from build123d import *

# Parameters (mm, degrees)
SKETCH_1_R               = 3
SKETCH_1_R_2             = 1.40625
EXTRUDE_1_DEPTH          = 5
CUT_EXTRUDE_2_DEPTH      = 7.557438524
PATTERN_CIRCULAR_1_COUNT = 7


with BuildPart() as part:
    # 草图1 → 凸台-拉伸1 (new body)
    with BuildSketch(Plane.XY):
        Circle(SKETCH_1_R)
        Circle(SKETCH_1_R_2, mode=Mode.SUBTRACT)
    extrude(amount=EXTRUDE_1_DEPTH)

    # 草图1<3> → 切除-拉伸2 (cut, through all)
    with BuildSketch(Plane.XY):
        with BuildLine():
            Line((1.546319716, 0.559598866), (1.322324253, 0.478536971))
            ThreePointArc((1.322324253, 0.478536971), (1.385109661, 0.242920339), (1.40625, 0))
            ThreePointArc((1.40625, 0), (1.385109661, -0.242920339), (1.322324253, -0.478536971))
            Line((1.322324253, -0.478536971), (1.546319716, -0.559598866))
            add(Edge.make_bspline(
                [(1.546319716, -0.559598866), (1.558105463, -0.563864019), (1.591921474, -0.573215837), (1.658734166, -0.580959295), (1.767731952, -0.57845396), (1.907008009, -0.553308364), (2.079413065, -0.496026363), (2.261035814, -0.40341458), (2.393734523, -0.311147352), (2.48335867, -0.236539754), (2.523284743, -0.200650618)],
                knots=[0, 0, 0, 0, 0, 0.005604068, 0.015718248, 0.029959916, 0.048733667, 0.068727063, 0.096888892, 0.120945025, 0.120945025, 0.120945025, 0.120945025, 0.120945025], degree=4))
            ThreePointArc((2.523284743, -0.200650618), (2.529257902, -0.100404327), (2.53125, 0))
            ThreePointArc((2.53125, 0), (2.529257902, 0.100404327), (2.523284743, 0.200650618))
            add(Edge.make_bspline(
                [(1.546319716, 0.559598866), (1.558105463, 0.563864019), (1.591921474, 0.573215837), (1.658734166, 0.580959295), (1.767731952, 0.57845396), (1.907008009, 0.553308364), (2.079413065, 0.496026363), (2.261035814, 0.40341458), (2.393734523, 0.311147352), (2.48335867, 0.236539754), (2.523284743, 0.200650618)],
                knots=[0, 0, 0, 0, 0, 0.005604068, 0.015718248, 0.029959916, 0.048733667, 0.068727063, 0.096888892, 0.120945025, 0.120945025, 0.120945025, 0.120945025, 0.120945025], degree=4))
        make_face()
    cut_extrude_2 = extrude(amount=CUT_EXTRUDE_2_DEPTH, mode=Mode.SUBTRACT)

    # 阵列(圆周)1: 切除-拉伸2 ×7 about axis
    pattern_circular_1_axis = Axis((0, 0, 5), (0, 0, 1))
    for i in range(1, PATTERN_CIRCULAR_1_COUNT):
        add(cut_extrude_2.rotate(pattern_circular_1_axis, i * 360 / PATTERN_CIRCULAR_1_COUNT), mode=Mode.SUBTRACT)


solid = part.part
Geometry check sheet. Reference: the model listing, model coordinates, mm. Coordinates: 2 decimals unless noted, no trailing zeros. Order: outer loops, then holes, each group sorted by start corner. A loop starts at its lowest first (then second) coordinate and runs counter-clockwise, first axis right, second up. Notation, with made-up numbers: (18.25, -20.5) -> (41.25, -20.5) arc R14 cw to (41.25, -14.5) -> close; hole circle Ø6 at (-1.75, 33). An arc over 180 degrees is marked (long way). Use a Markdown table: item, result. Add a question column.
1. Cross-section at C-C (x = 2.75). Enter the section's corners in (y, z), and give its area (3 significant figures).
2. Go/stop test with flat-tipped pins: pin 1 Ø3 at (y, z) = (2, 3.5) entering from -X; pin 2 Ø1.5 at (x, z) = (-2, 1) entering from +Y. Record where each tip stops, or that it passes through.
3. Cross-section at A-A (y = 1.75). Give the number of separate pieces and of enclosed holes in the cut face, and give its area (3 significant figures).
4. Material ranges on L1, parallel to X at y = 1.5, z = 4.6; L2, parallel to Y at x = 1, z = 3.45; L3, parallel to Y at x = -0.5, z = 0.7, recorded low to high.
Filled sheet:
| question | item | result |
|---|---|---|
| 1 | outline | (-1.2, 0) -> (1.2, 0) -> (1.2, 5) -> (-1.2, 5) -> close |
| 1 | area | 12.0 mm2 |
| 2 | pin 1 | x = -2.96 |
| 2 | pin 2 | y = 2.73 |
| 3 | separate pieces | 3 |
| 3 | enclosed holes | 0 |
| 3 | area | 13.3 mm2 |
| 4 | L1 | -2.6 to -0.94, 0.19 to 0.51, 1.72 to 2.6 |
| 4 | L2 | -2.83 to -1.97, 1.97 to 2.83 |
| 4 | L3 | -2.96 to -2.48, 2.48 to 2.96 |
